Autodesk Inventor part; units mm, degrees
ref_plane "YZ Plane" through (0, 0, 0) normal (1, 0, 0) x (0, 1, 0)
ref_plane "XZ Plane" through (0, 0, 0) normal (0, 1, 0) x (-1, 0, 0)
ref_plane "XY Plane" through (0, 0, 0) normal (0, 0, 1) x (1, 0, 0)
sketch "Sketch1" plane through (0, 0, 0) normal (0, 1, 0) x (-1, 0, 0)
  line L0 (-20.2311, -10.16) -> (20.2311, -10.16)
  line L1 (20.2311, -10.16) -> (20.2311, 10.16)
  line L2 (20.2311, 10.16) -> (-20.2311, 10.16)
  line L3 (-20.2311, 10.16) -> (-20.2311, -10.16)
  line L4 (-20.2311, -10.16) -> (20.2311, 10.16) construction
  line L5 (20.2311, -10.16) -> (-20.2311, 10.16) construction
  point P0 (0, 0)
  dimension "d0" = 40.4622
  dimension "d1" = 20.32
extrude "Extrusion1" add sketch "Sketch1" along normal blind 36.068
sketch "Sketch2" plane through (0, 36.068, 0) normal (0, 1, 0) x (1, 0, 0)
  line L0 (-20.2311, -10.16) -> (20.2311, -10.16)
  line L1 (20.2311, -10.16) -> (20.2311, 10.16)
  circle A0 centre (10.0711, 0) radius 6.985
  circle A1 centre (10.0711, 0) radius 5.08
  point P0 (0, 0)
  dimension "d4" = 13.97
  dimension "d5" = 10.16
  dimension "d6" = 10.16
  dimension "d7" = 10.16
extrude "Extrusion2" add sketch "Sketch2" along normal blind 2.032 contours A1
chamfer "Chamfer1" distance 1.9812 angle 45 1 edges at (4.9911, 36.068, 0)
sketch "Sketch3" plane through (10.0711, 38.1, 0) normal (0, 1, 0) x (1, 0, 0)
  circle A0 centre (0, 0) radius 5.08
  point P0 (-10.0711, 0)
ref_plane "Work Plane1" through (0, 38.1, 0) normal (1, 0, 0) x (0, 0, -1)
sketch "Sketch4" plane through (20.2311, 0, 10.16) normal (1, 0, 0) x (0, 0, -1)
  line L0 (20.32, 0) -> (20.32, 36.068)
  line L1 (0, 36.068) -> (20.32, 36.068)
  line L2 (20.32, 36.068) -> (20.32, 30.48)
  line L3 (20.32, 30.48) -> (0, 30.48)
  line L4 (0, 30.48) -> (0, 36.068)
  line L5 (0, 30.48) -> (20.32, 30.48)
  line L6 (20.32, 30.48) -> (20.32, 24.638)
  line L7 (20.32, 24.638) -> (0, 24.638)
  line L8 (0, 24.638) -> (0, 30.48)
  point P0 (10.16, 0)
  dimension "d14" = 5.588
  dimension "d16" = 5.842
extrude "Extrusion3" add sketch "Sketch4" along normal blind 8.636 contours L7 L8 L3 L0
sketch "Sketch5" plane through (20.2311, 30.48, 10.16) normal (0, 1, 0) x (1, 0, 0)
  line L0 (0, 0) -> (8.636, 0)
  line L1 (8.636, 20.32) -> (8.636, 0)
  line L2 (0, 20.32) -> (8.636, 20.32)
  point P0 (-20.2311, 10.16)
  point P1 (4.7752, 16.4592)
  point P2 (4.7752, 3.8608)
  dimension "d19" = 3.8608
  dimension "d20" = 3.8608
  dimension "d21" = 3.8608
  dimension "d22" = 3.8608
hole "Hole1" at (25.0063, 30.48, -6.2992) at (25.0063, 30.48, 6.2992) direction (0, -1, 0) diameter 2.7686 end through all
mirror "Mirror1" about plane through (0, 38.1, 0) normal (1, 0, 0) of "Extrusion3", "Hole1"
sketch "Sketch6" plane through (20.2311, 0, 10.16) normal (1, 0, 0) x (0, 0, -1)
  line L0 (20.32, 24.638) -> (0, 24.638)
  line L1 (0, 0) -> (0, 24.638)
  line L2 (0, 0) -> (20.32, 0)
  line L3 (20.32, 0) -> (20.32, 24.638)
  line L4 (5.7791, 2.54) -> (13.4355, 2.54)
  point P0 (10.16, 0)
  point P1 (10.16, 2.54)
  point P2 (10.922, 2.54)
  point P3 (9.398, 2.54)
  dimension "d30" = 0.762
  dimension "d32" = 0.762
  dimension "d33" = 0
  dimension "d34" = 2.54
properties material "Aluminum 6061"
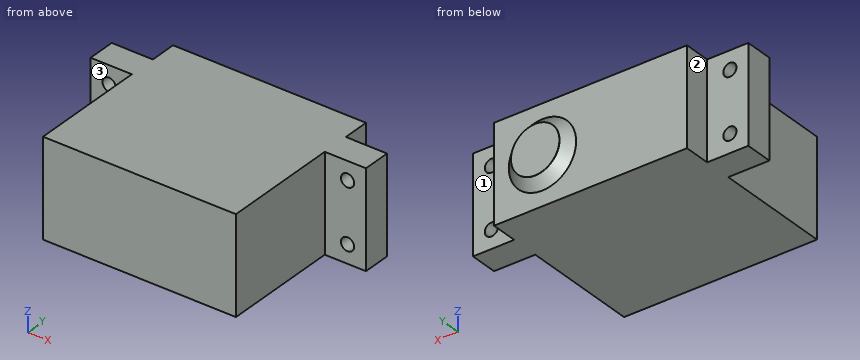
Can you work these out from the model? Positions are in its coordinate system, mm. Face numbers are marked on the shaded views. A direction names the side the tool comes from. Coordinates: 2 decimals unless noted, no trailing zeros. Write each loop counter-clockwise with the first axis right and the second up, starting at its lowest first coordinate (ties: lowest second). Pieces come first, ordered by that corner, then holes. Notation, with made-up numbers: (79.5, 82) - (132.5, 82) arc R14 cw to (132.5, 91) - close; hole circle Ø6 at (16, 54.25). An arc over 180 degrees is marked (long way). Return JSON: item names as keys, results as strings. Group by question number.
Item 1: I'm going to push flat-ended pins straight in: pin 1 Ø4.5 at (x, z) = (-26.5, -4.5) entering from -Y; pin 2 Ø1 at (y, z) = (10, -8) entering from +X; pin 3 Ø2.5 at (x, z) = (26.5, -4.5) entering from +Y. Where does each tip first touch, or does it pass through?
Item 2: Please list where these lines run through material, in increasing order: probe 1 along X at (y, z) = (27, 6.25); probe 2 along X at (y, z) = (24, -8.75); probe 3 along Y at (x, z) = (22, 1.75).
Item 3: If we section it at A-A (z = 0): Write out the boundary of the cut face in (x, y).
Item 4: If we section it at B-B (y = 29): Write out the boundary of the cut face in (x, z).
Item 5: If we section it at C-C (z = 8.5): Write out the boundary of the cut face in (x, y).
Item 6: If we section it at D-D (x = -21.5): Write out the boundary of the cut face in (y, z).
Item 7: Which directions (+Z, -Z, +X, -X, +Y, -Y) give clear straight access to the entire face, cutting with the end or side of a thin tool? Please do the marked faces 1, 2 and 3.
Return value:
{
 "1": {"pin 1": "stops at y = 24.64", "pin 2": "stops at x = 20.23", "pin 3": "stops at y = 30.48"},
 "2": {"probe 1": "x = -28.87 to -26.39, -23.62 to 23.62, 26.39 to 28.87", "probe 2": "x = -20.23 to 20.23", "probe 3": "y = 24.64 to 30.48"},
 "3": {"outline": "(-28.87, 24.64) - (-20.23, 24.64) - (-20.23, 0) - (20.23, 0) - (20.23, 24.64) - (28.87, 24.64) - (28.87, 30.48) - (20.23, 30.48) - (20.23, 36.07) - (17.13, 36.07) - (15.15, 38.05) - (15.15, 38.1) - (4.99, 38.1) - (4.99, 38.05) - (3.01, 36.07) - (-20.23, 36.07) - (-20.23, 30.48) - (-28.87, 30.48) - close"},
 "4": {"outline": "(-28.87, -10.16) - (28.87, -10.16) - (28.87, 10.16) - (-28.87, 10.16) - close; hole circle Ø2.77 at (-25.01, -6.3); hole circle Ø2.77 at (-25.01, 6.3); hole circle Ø2.77 at (25.01, -6.3); hole circle Ø2.77 at (25.01, 6.3)"},
 "5": {"outline": "(-28.87, 24.64) - (-20.23, 24.64) - (-20.23, 0) - (20.23, 0) - (20.23, 24.64) - (28.87, 24.64) - (28.87, 30.48) - (20.23, 30.48) - (20.23, 36.07) - (-20.23, 36.07) - (-20.23, 30.48) - (-28.87, 30.48) - close"},
 "6": {"outline": "(24.64, -10.16) - (30.48, -10.16) - (30.48, 10.16) - (24.64, 10.16) - close"},
 "7": {"face 1": "+Z, -Z, +X, +Y", "face 2": "+Z, -Z, -X, +Y", "face 3": "+Z, -Z, -X, -Y"}
}
